Read the model definition and answer for the solid it produces. Units are mm, in the model's axes. Give positions to 0.01 mm unless a question says otherwise; leave off trailing zeros. Write each loop counter-clockwise with the first axis right and the second up, starting at its lowest first coordinate (ties: lowest second). Pieces come first, ordered by that corner, then holes. Notation, with made-up numbers: M -16.5,43 L 41.5,43 A31 cw 41.5,74 Z; hole C 12,-27.75 d3. An arc over 180 degrees is marked long. Answer as CSV lines item,"result". Start each with the question number.
```python
from build123d import *

# Parameters (mm, degrees)
BOSS_EXTRUDE4_DEPTH = 6


with BuildPart() as part:
    # Sketch2 → Boss-Extrude4 (new body)
    with BuildSketch(Plane.XY):
        Polygon((45, 9.865384615), (3, 9.865384615), (3, 54.865384615), (-3, 54.865384615), (-3, 9.865384615), (-45, 9.865384615), (-22.5, 99.865384615), (-15.25, 99.865384615), (-15.25, 105.865384615), (-7.25, 105.865384615), (-7.25, 99.865384615), (7.25, 99.865384615), (7.25, 105.865384615), (15.25, 105.865384615), (15.25, 99.865384615), (22.5, 99.865384615), align=None)
        Polygon((-8, 94.865384615), (-18.596117968, 94.865384615), (-38.596117968, 14.865384615), (-8, 14.865384615), align=None, mode=Mode.SUBTRACT)
        Polygon((38.596117968, 14.865384615), (8, 14.865384615), (8, 94.865384615), (18.596117968, 94.865384615), align=None, mode=Mode.SUBTRACT)
    extrude(amount=BOSS_EXTRUDE4_DEPTH)


solid = part.part
```
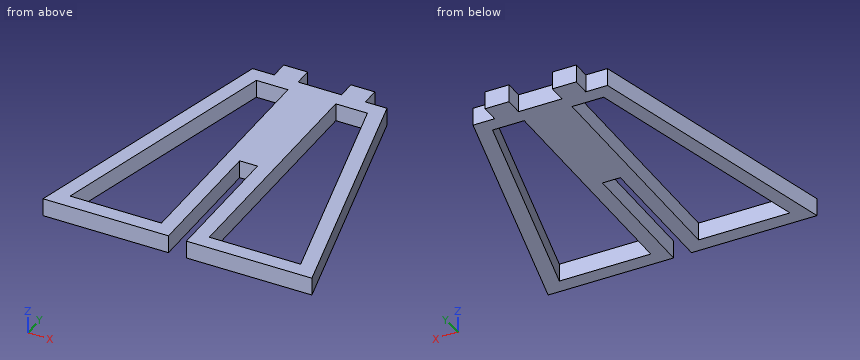
1. Find the intervals of material crossed by line 1 (X direction, y = 44.5, z = 5.5); line 2 (X direction, y = 16.5, z = 2.85); line 3 (X direction, y = 61.5, z = 4.6), in increasing order. Write a range as [from, to].
2. Find section C-C on y = 74. Determine the outline of the cut face in (x, z), then the cut area to 3 significant figures.
3. Find section A-A on z = 2.3. Determine the outline of the cut face in (x, y), then the cut area to 3 significant figures.
4. Find section B-B on x = -9.5. Determine the outline of the cut face in (y, z).
5. Given pin 1 (3 mm diameter, centred on y = 104, z = 4.5, fed in from -X); pin 2 (2 mm diameter, centred on x = -23, z = 3.5, fed in from +Y); pin 3 (12 mm diameter, centred on x = 24.5, y = 23, fed in from -Z); pin 4 (1.8 mm diameter, centred on x = -0.5, z = 3, fed in from -Y), each flat-ended and moving along its own axis, determine where each tip first touches the part or whether it passes through.
6. Find section D-D on y = 49. Determine the outline of the cut face in (x, z), then the cut area to 3 significant figures.
Computed:
1,line 1,"x = [-36.34, -31.19], [-8, -3], [3, 8], [31.19, 36.34]"
1,line 2,"x = [-43.34, -38.19], [-8, -3], [3, 8], [38.19, 43.34]"
1,line 3,"x = [-32.09, -26.94], [-8, 8], [26.94, 32.09]"
2,outline,"M -28.97,0 L -23.81,0 L -23.81,6 L -28.97,6 Z; M -8,0 L 8,0 L 8,6 L -8,6 Z; M 23.81,0 L 28.97,0 L 28.97,6 L 23.81,6 Z"
2,area,"158 mm^2"
3,outline,"M -45,9.87 L -3,9.87 L -3,54.87 L 3,54.87 L 3,9.87 L 45,9.87 L 22.5,99.87 L 15.25,99.87 L 15.25,105.87 L 7.25,105.87 L 7.25,99.87 L -7.25,99.87 L -7.25,105.87 L -15.25,105.87 L -15.25,99.87 L -22.5,99.87 Z; hole M -38.6,14.87 L -8,14.87 L -8,94.87 L -18.6,94.87 Z; hole M 8,14.87 L 38.6,14.87 L 18.6,94.87 L 8,94.87 Z"
3,area,"2,610 mm^2"
4,outline,"M 9.87,0 L 14.87,0 L 14.87,6 L 9.87,6 Z; M 94.87,0 L 105.87,0 L 105.87,6 L 94.87,6 Z"
5,pin 1,"stops at x = -15.25"
5,pin 2,"stops at y = 99.87"
5,pin 3,"passes through"
5,pin 4,"stops at y = 54.87"
6,outline,"M -35.22,0 L -30.06,0 L -30.06,6 L -35.22,6 Z; M -8,0 L -3,0 L -3,6 L -8,6 Z; M 3,0 L 8,0 L 8,6 L 3,6 Z; M 30.06,0 L 35.22,0 L 35.22,6 L 30.06,6 Z"
6,area,"122 mm^2"
